Design review of the part built by this model. Coordinates are the model's own, in mm. A direction names the side the tool comes from. Coordinates: 2 decimals unless noted, no trailing zeros. Loops run counter-clockwise (first coordinate to the right, second up) from the corner with the lowest first, then second, coordinate; pieces in that order, holes last.
from build123d import *

# Parameters (mm, degrees)
BOSS_EXTRUDE1_DEPTH = 100
SKETCH2_R           = 2.5
CUT_EXTRUDE1_DEPTH  = 225.499443206


with BuildPart() as part:
    # Sketch1 → Boss-Extrude1 (new, symmetric)
    with BuildSketch(Plane.XY):
        Polygon((0, 20), (0, 0), (200, 0), (200, 20), (198, 20), (198, 2), (2, 2), (2, 20), align=None)
    extrude(amount=BOSS_EXTRUDE1_DEPTH, both=True)

    # Sketch2 → Cut-Extrude1 (cut, through all)
    with BuildSketch(Plane(origin=(200, 0, 0), x_dir=(0, 0, -1), z_dir=(1, 0, 0))):
        with Locations((-85, 10)):
            Circle(SKETCH2_R)
        with BuildLine():
            Line((70, 7.5), (-10, 7.5))
            ThreePointArc((-10, 7.5), (-12.5, 10), (-10, 12.5))
            Line((-10, 12.5), (70, 12.5))
            ThreePointArc((70, 12.5), (72.5, 10), (70, 7.5))
        make_face()
    extrude(amount=-CUT_EXTRUDE1_DEPTH, mode=Mode.SUBTRACT)


solid = part.part
Q1. Take a section at B-B, the plane z = 1. Write out the cut boundary in (x, y).
Q2. The part is to be moulded in two halves that separate along X. For faces 1 (the flat face through (0, 6, 1)), 2 (the flat face through (100, 1, 100)), 3 (the flat face through (198, 13, 1)), say which applies: pulls with the +X half, pulls with the -X half, needs draft (parallel to the pull), parting line crosses it, or undercut.
Q3. Take a section at A-A, the plane y = 10. Write out the cut boundary in (x, z), then the cut area to 3 significant figures.
Q4. Machinability: for faces 4 (the cylindrical face through (1, 8.5, 87)), 5 (the flat face through (2, 13, 1)), which of the approach directions +Z, -Z, +X, -X, +Y, -Y give a long, thin tool a straight path to every point of the face, cutting with its end or side? Answer none if there is none.
Q5. Take a section at C-C, the plane z = 27. Write out the cut boundary in (x, y).
Q6. For line 1 (Y direction, x = 0.5, z = 85); line 2 (X direction, y = 5.5, z = 57); line 3 (Y direction, x = 64.5, z = -81), list the stretches that pass through material, from the lowest coordinate up.
Q7. Take a section at D-D, the plane x = 42.5. Write out the cut boundary in (y, z), then the cut area to 3 significant figures.
Q8. Clearance check with a flat-ended pin moving along its axis: pin 1 Ø4 at (x, z) = (24.5, -17.5) entering from +Y. State where the tip first meets the part, or that it passes through.
Entries:
1. outline: (0, 0) - (200, 0) - (200, 7.5) - (198, 7.5) - (198, 2) - (2, 2) - (2, 7.5) - (0, 7.5) - close; (0, 12.5) - (2, 12.5) - (2, 20) - (0, 20) - close; (198, 12.5) - (200, 12.5) - (200, 20) - (198, 20) - close
2. face 1: pulls with the -X half
2. face 2: needs draft
2. face 3: undercut
3. outline: (0, -100) - (2, -100) - (2, -72.5) - (0, -72.5) - close; (0, 12.5) - (2, 12.5) - (2, 82.5) - (0, 82.5) - close; (0, 87.5) - (2, 87.5) - (2, 100) - (0, 100) - close; (198, -100) - (200, -100) - (200, -72.5) - (198, -72.5) - close; (198, 12.5) - (200, 12.5) - (200, 82.5) - (198, 82.5) - close; (198, 87.5) - (200, 87.5) - (200, 100) - (198, 100) - close
3. area: 440 mm2
4. face 4: +X, -X
4. face 5: +Z, -Z, +Y
5. outline: (0, 0) - (200, 0) - (200, 20) - (198, 20) - (198, 2) - (2, 2) - (2, 20) - (0, 20) - close
6. line 1: y = 0 to 7.5, 12.5 to 20
6. line 2: x = 0 to 2, 198 to 200
6. line 3: y = 0 to 2
7. outline: (0, -100) - (2, -100) - (2, 100) - (0, 100) - close
7. area: 400 mm2
8. pin 1: stops at y = 2
